from build123d import *

# Parameters (mm, degrees)
RESSALTO_EXTRUS_O1_DEPTH = 10
ESBO_O2_OUTSIDE_W        = 140.39
ESBO_O2_OUTSIDE_H        = 143.484
ESBO_O2_OUTSIDE_R        = 10
CORTE_EXTRUS_O1_DEPTH    = 15
CORTE_EXTRUS_O1_DRAFT    = -75
ESBO_O3_OUTSIDE_W        = 140.39
ESBO_O3_OUTSIDE_H        = 143.484
ESBO_O3_OUTSIDE_R        = 10
CORTE_EXTRUS_O2_DEPTH    = 15
CORTE_EXTRUS_O2_DRAFT    = -75
FURO_ROSCADO_DE_M121_D   = 10.2
CHANFRO3_SIZE            = 0.5
CHANFRO4_SIZE            = 0.5


with BuildPart() as part:
    # Esboço1 → Ressalto-extrusão1 (new body)
    with BuildSketch(Plane.XY):
        Polygon((0, 11.547005384), (-10, 5.773502692), (-10, -5.773502692), (0, -11.547005384), (10, -5.773502692), (10, 5.773502692), align=None)
    extrude(amount=RESSALTO_EXTRUS_O1_DEPTH)


with BuildPart() as corte_extrus_o1_tool:
    # Esboço2 outside → Corte-extrusão1 (with draft: the straight prism first)
    with BuildSketch(Plane.XY.offset(10)):
        Rectangle(ESBO_O2_OUTSIDE_W, ESBO_O2_OUTSIDE_H)
        Circle(ESBO_O2_OUTSIDE_R, mode=Mode.SUBTRACT)
    extrude(amount=-CORTE_EXTRUS_O1_DEPTH)
    # Corte-extrusão1: the draft: its side faces are tilted about the plane it starts from
    corte_extrus_o1_sides = [corte_extrus_o1_tool.faces().sort_by_distance(p)[0] for p in [
        (0, -71.742, 2.5),
        (70.195, 0, 2.5),
        (0, 71.742, 2.5),
        (-70.195, 0, 2.5),
        (-10, 0, 2.5),
    ]]
    draft(corte_extrus_o1_sides, Plane.XY.offset(10), CORTE_EXTRUS_O1_DRAFT)


with BuildPart() as part_1:
    add(part.part)

    # Corte-extrusão1: cut by corte_extrus_o1_tool
    add(corte_extrus_o1_tool.part, mode=Mode.SUBTRACT)


with BuildPart() as corte_extrus_o2_tool:
    # Esboço3 outside → Corte-extrusão2 (with draft: the straight prism first)
    with BuildSketch(Plane(origin=(0, 0, 0), x_dir=(-1, 0, 0), z_dir=(0, 0, -1))):
        Rectangle(ESBO_O3_OUTSIDE_W, ESBO_O3_OUTSIDE_H)
        Circle(ESBO_O3_OUTSIDE_R, mode=Mode.SUBTRACT)
    extrude(amount=-CORTE_EXTRUS_O2_DEPTH)
    # Corte-extrusão2: the draft: its side faces are tilted about the plane it starts from
    corte_extrus_o2_sides = [corte_extrus_o2_tool.faces().sort_by_distance(p)[0] for p in [
        (0, -71.742, 7.5),
        (-70.195, 0, 7.5),
        (0, 71.742, 7.5),
        (70.195, 0, 7.5),
        (10, 0, 7.5),
    ]]
    draft(corte_extrus_o2_sides, Plane(origin=(0, 0, 0), x_dir=(-1, 0, 0), z_dir=(0, 0, -1)), CORTE_EXTRUS_O2_DRAFT)


with BuildPart() as part_2:
    add(part_1.part)

    # Corte-extrusão2: cut by corte_extrus_o2_tool
    add(corte_extrus_o2_tool.part, mode=Mode.SUBTRACT)

    # Furo roscado de M121 (through all)
    with Locations(Plane(origin=(0, 0, 0), x_dir=(-1, 0, 0), z_dir=(0, 0, -1))):
        with Locations((0, 0)):
            Hole(FURO_ROSCADO_DE_M121_D / 2)

    # Chanfro3
    chanfro3_edges = [part_2.edges().sort_by_distance(p)[0] for p in [
        (-5.1, 0, 10),
    ]]
    chamfer(chanfro3_edges, length=CHANFRO3_SIZE)

    # Chanfro4
    chanfro4_edges = [part_2.edges().sort_by_distance(p)[0] for p in [
        (-5.1, 0, 0),
    ]]
    chamfer(chanfro4_edges, length=CHANFRO4_SIZE)


solid = part_2.part
The model under review builds one solid part; all positions refer to its coordinate system, in mm. Give positions to 0.01 mm unless a question says otherwise; leave off trailing zeros. Loops run counter-clockwise (first coordinate to the right, second up) from the corner with the lowest first, then second, coordinate; pieces in that order, holes last. Notation, with made-up numbers: (34, -35.5) -> (53, -35.5) arc R28 cw to (53, -3.5) -> close; hole circle Ø5 at (49.25, 38). An arc over 180 degrees is marked (long way). Answer as a JSON object with one key per item and string values. Group by question number.
Q1. Take a section at A-A (z = 1.5). Write out the cut boundary in (x, y), plus the area to 3 significant figures.
Q2. Insertion check: pin 1 (1 mm diameter, centred on y = 9, z = 6, fed in from +X); pin 2 (1 mm diameter, centred on x = 7, z = 1.5, fed in from -Y); pin 3 (1.5 mm diameter, centred on x = -7.5, z = 7.5, fed in from -Y). Each pin has a flat end and moves straight along its axis. Give the tip position at first contact, or say it passes through.
Q3. Wall thickness on line 1 along X through (y, z) = (-2.25, 6.5); line 2 along Y through (x, z) = (-3.5, 5.75); line 3 along X through (y, z) = (-3.25, 3.75): over which ranges is each line inside the solid? List them lowest first.
Answer below:
{
 "1": {"outline": "(-10, -5.77) -> (0, -11.55) -> (10, -5.77) -> (10, 5.77) -> (0, 11.55) -> (-10, 5.77) -> close; hole circle Ø10.2 at (0, 0)", "area": "265 mm2"},
 "2": {"pin 1": "stops at x = 5.28", "pin 2": "stops at y = -7.79", "pin 3": "stops at y = -7.65"},
 "3": {"line 1": "x = -10 to -4.58, 4.58 to 10", "line 2": "y = -9.53 to -3.71, 3.71 to 9.53", "line 3": "x = -10 to -3.93, 3.93 to 10"}
}
